from build123d import *

# Parameters (mm, degrees)
F0_W      = 74.6125
F0_H      = 19.05
F1_DEPTH  = 342.9
F2_W      = 25.4
F2_H      = 19.05
F3_DEPTH  = 381
F4_W      = 44.45
F4_H      = 19.05
F5_DEPTH  = 330.2
F6_W      = 6.35
F6_H      = 19.05
F6_W_2    = 0.79375
F6_H_2    = 9.525
F6_W_3    = 42.8625
F7_DEPTH  = 330.2
F9_D      = 9.525
F9_DEPTH  = 19.051
F10_W     = 9.504689079
F10_H     = 254.1668581462
F11_DEPTH = 19.051
F13_D     = 3.175


with BuildPart() as f1:
    # F0 (on Top) → F1 (new body, symmetric)
    with BuildSketch(Plane.XY):
        Rectangle(F0_W, F0_H)
    extrude(amount=F1_DEPTH, both=True)

    # F2 (on face) → F3 (join)
    with BuildSketch(Plane(origin=(0, 0, -342.9), x_dir=(1, 0, 0), z_dir=(0, 0, -1))):
        with Locations((0, -9.525)):
            Rectangle(F2_W, F2_H)
    extrude(amount=-F3_DEPTH)

    # F4 (on face) → F5 (cut)
    with BuildSketch(Plane.XY.offset(342.9)):
        with Locations((0, -9.525)):
            Rectangle(F4_W, F4_H)
    extrude(amount=-F5_DEPTH, mode=Mode.SUBTRACT)

    # F6 (on face) → F7 (cut)
    with BuildSketch(Plane(origin=(0, 0, -342.9), x_dir=(1, 0, 0), z_dir=(0, 0, -1))):
        with Locations((-34.13125, 0)):
            Rectangle(F6_W, F6_H)
        Polygon((-30.95625, 9.525), (-30.95625, -9.525), (-21.43125, -9.525), (-21.43125, 0), (-22.225, 0), (-22.225, 9.525), align=None)
        with Locations((-21.828125, 4.7625)):
            Rectangle(F6_W_2, F6_H_2)
        with Locations((0, 4.7625)):
            Rectangle(F6_W_3, F6_H_2)
        Polygon((22.225, 0), (21.43125, 0), (21.43125, -9.525), (30.95625, -9.525), (30.95625, 9.525), (22.225, 9.525), align=None)
        with Locations((21.828125, 4.7625)):
            Rectangle(F6_W_2, F6_H_2)
        with Locations((34.13125, 0)):
            Rectangle(F6_W, F6_H)
    extrude(amount=-F7_DEPTH, mode=Mode.SUBTRACT)

    # F9 (through all, one way)
    with BuildSketch(Plane(origin=(0, 9.525, 0), x_dir=(-1, 0, 0), z_dir=(0, 1, 0))):
        with Locations((0, -317.5), (0, -215.9), (0, -114.3), (0, 50.8), (0, 304.8)):
            Circle(F9_D / 2)
    extrude(amount=-F9_DEPTH, mode=Mode.SUBTRACT)

    # F10 (on face) → F11 (cut, through all)
    with BuildSketch(Plane(origin=(0, 9.525, 0), x_dir=(-1, 0, 0), z_dir=(0, 1, 0))):
        with Locations((-0.0052560493, 177.5006012835)):
            Rectangle(F10_W, F10_H)
    extrude(amount=-F11_DEPTH, mode=Mode.SUBTRACT)

    # F13 (through all)
    with Locations(Plane(origin=(-37.30625, 0, 0), x_dir=(0, -1, 0), z_dir=(-1, 0, 0))):
        with Locations((0, 317.5), (0, 0)):
            Hole(F13_D / 2)


solid = f1.part
For this review, take the finished solid that the model builds, in its own axes (mm). A direction names the side the tool comes from. Coordinates: 2 decimals unless noted, no trailing zeros. Loops run counter-clockwise (first coordinate to the right, second up) from the corner with the lowest first, then second, coordinate; pieces in that order, holes last. Notation, with made-up numbers: (87, -1.5) - (126, -1.5) arc R7 ccw to (126, 2.5) - close; hole circle Ø11 at (79.25, 61.5). An arc over 180 degrees is marked (long way). Use a Markdown table: item, result. Add a question column.
Item 1: Mouldability with a two-part tool opening along X and no side actions: class faces 4 (the face through (0, 7, -342.9)), 5 (the face through (37.306, 0, 168)), 6 (the face through (0, 0, 331)), 7 (the face through (-37.306, 0, 168)) as pulls with the +X half, pulls with the -X half, needs draft (parallel to the pull), parting line crosses it, or undercut.
Item 2: For line 1 (Z direction, x = 0, y = 2.25); line 2 (X direction, y = -3, z = 141.5) (3 decimals); line 3 (X direction, y = 7, z = 181), list the stretches that pass through material, from the lowest coordinate up.
Item 3: We need section B-B (z = -22). Give the boundary of the cut face in (x, y) (3 decimals).
Item 4: Insertion check: pin 1 Ø21.5 at (x, z) = (8, -150.5) entering from -Y; pin 2 Ø12 at (x, z) = (-22, 245) entering from -Y (3 decimals); pin 3 Ø3 at (y, z) = (13, -225.5) entering from +X; pin 4 Ø7.5 at (x, z) = (0, -114.3) entering from -Y (3 decimals). Each pin has a flat end and moves straight along its axis. Give the tip position at first contact, or say it passes through.
Item 5: Tool access review of faces 1 (the face through (-5, 0, 166)), 2 (the face through (0, 0, -180)), 3 (the face through (-1, 2, 342.9)): name each direction out of +Z, -Z, +X, -X, +Y, -Y from which nothing blocks a thin tool from reaching the whole face with its end or side.
Item 6: We need section A-A (z = 215). Give the boundary of the cut face in (x, y) (3 decimals).
Results list:
| question | item | result |
|---|---|---|
| 1 | face 4 | needs draft |
| 1 | face 5 | pulls with the +X half |
| 1 | face 6 | undercut |
| 1 | face 7 | pulls with the -X half |
| 2 | line 1 | z = -342.9 to -322.26, -312.74 to -220.66, -211.14 to -119.06, -109.54 to 46.04, 309.56 to 342.9 |
| 2 | line 2 | x = -37.306 to -22.225, 22.225 to 37.306 |
| 2 | line 3 | x = -37.31 to -4.75, 4.76 to 37.31 |
| 3 | outline | (-21.431, 0) - (21.431, 0) - (21.431, 9.525) - (12.7, 9.525) - (12.7, 19.05) - (-12.7, 19.05) - (-12.7, 9.525) - (-21.431, 9.525) - close |
| 4 | pin 1 | stops at y = 0 |
| 4 | pin 2 | stops at y = -9.525 |
| 4 | pin 3 | stops at x = 12.7 |
| 4 | pin 4 | stops at y = 9.525 |
| 5 | face 1 | +Z, -Y |
| 5 | face 2 | -Z, +X, -X, -Y |
| 5 | face 3 | +Z, +X, -X, +Y, -Y |
| 6 | outline | (-37.306, -9.525) - (-22.225, -9.525) - (-22.225, 0) - (-4.747, 0) - (-4.747, 9.525) - (-37.306, 9.525) - close; (4.758, 0) - (22.225, 0) - (22.225, -9.525) - (37.306, -9.525) - (37.306, 9.525) - (4.758, 9.525) - close |
